```python
from build123d import *

# Parameters (mm, degrees)
F0_W          = 324
F0_H          = 18
F1_DEPTH      = 115
F2_DEPTH      = 130
F2_DEPTH_BACK = 10
F3_SIZE       = 8
F0_H_2        = 692
F4_DEPTH      = 4


with BuildPart() as f1:
    # F0 (on Top) → F1 (new body)
    with BuildSketch(Plane.XY):
        Polygon((162, 710), (162, 18), (180, 18), (180, 728), (162, 728), align=None)
        with Locations((0, 719)):
            Rectangle(F0_W, F0_H)
        Polygon((-180, 728), (-180, 18), (-162, 18), (-162, 710), (-162, 728), align=None)
    extrude(amount=F1_DEPTH)

    # F0 (on Top) → F2 (join, two sides)
    with BuildSketch(Plane.XY) as f2_sk:
        Polygon((-162, 18), (-180, 18), (-200, 18), (-200, 0), (200, 0), (200, 18), (180, 18), (162, 18), align=None)
    extrude(amount=F2_DEPTH)
    extrude(f2_sk.sketch, amount=-F2_DEPTH_BACK)

    # F3
    f3_edges = [f1.edges().sort_by_distance(p)[0] for p in [
        (0, 18, 130),
    ]]
    chamfer(f3_edges, length=F3_SIZE)

    # F0 (on Top) → F4 (join)
    with BuildSketch(Plane.XY):
        with Locations((0, 364)):
            Rectangle(F0_W, F0_H_2)
    extrude(amount=F4_DEPTH)


solid = f1.part
```
Part model, mm, in its own coordinate system. A direction names the side the tool comes from. Round coordinates to 2 decimals unless told otherwise and drop trailing zeros. Loops run counter-clockwise (first coordinate to the right, second up) from the corner with the lowest first, then second, coordinate; pieces in that order, holes last. Notation, with made-up numbers: (51, 5.5) -> (70, 5.5) arc R19 cw to (70, 25.5) -> close; hole circle Ø9 at (23, 35.5). An arc over 180 degrees is marked (long way). Use a Markdown table: item, result.
1) Cut at A-A, the plane z = 26. List the corners of the cut face in (x, y), and give its area (3 significant figures).
The answers:
| item | result |
|---|---|
| outline | (-200, 0) -> (200, 0) -> (200, 18) -> (180, 18) -> (180, 728) -> (-180, 728) -> (-180, 18) -> (-200, 18) -> close; hole (-162, 18) -> (162, 18) -> (162, 710) -> (-162, 710) -> close |
| area | 38,600 mm2 |
2) Drop flat-ended pins along their axis: pin 1 Ø10 at (x, y) = (100, 189) entering from -Z; pin 2 Ø1.5 at (x, y) = (-96.5, 480.5) entering from +Z; pin 3 Ø5 at (y, z) = (271, 91.5) entering from -X. Give the stop position or say it passes through.
The answers:
| item | result |
|---|---|
| pin 1 | stops at z = 0 |
| pin 2 | stops at z = 4 |
| pin 3 | stops at x = -180 |
3) Pull direction Y, two halves, no side cores. Call faces 1 (the flat face through (-3, 0, 61)), 2 (the flat face through (3, 18, 57)), 3 (the flat face through (-3, 378, 0)): pulls with the +Y half, pulls with the -Y half, needs draft (parallel to the pull), parting line crosses it, or undercut.
The answers:
| item | result |
|---|---|
| face 1 | pulls with the -Y half |
| face 2 | undercut |
| face 3 | needs draft |
4) Cut at C-C, the plane y = 51. List the corners of the cut face in (x, z), and give its area (3 significant figures).
The answers:
| item | result |
|---|---|
| outline | (-180, 0) -> (180, 0) -> (180, 115) -> (162, 115) -> (162, 4) -> (-162, 4) -> (-162, 115) -> (-180, 115) -> close |
| area | 5,440 mm2 |
5) Cut at B-B, the plane x = 7. List the corners of the cut face in (y, z), and give its area (3 significant figures).
The answers:
| item | result |
|---|---|
| outline | (0, -10) -> (18, -10) -> (18, 0) -> (728, 0) -> (728, 115) -> (710, 115) -> (710, 4) -> (18, 4) -> (18, 122) -> (10, 130) -> (0, 130) -> close |
| area | 7,330 mm2 |
6) Tool access for faces 4 (the flat face through (-174, 480, 115)), 5 (the flat face through (-180, 378, 57)), 6 (the flat face through (200, 9, 61)), 7 (the flat face through (180, 368, 57)), 8 (the flat face through (162, 369, 59)): list every direction of +Z, -Z, +X, -X, +Y, -Y with a clear straight run to the whole face (end or side of a thin tool).
The answers:
| item | result |
|---|---|
| face 4 | +Z, +X, -X, +Y |
| face 5 | +Z, -Z, -X, +Y |
| face 6 | +Z, -Z, +X, +Y, -Y |
| face 7 | +Z, -Z, +X, +Y |
| face 8 | +Z |
7) Probe line 1 (X direction, y = 531.5, z = 55); line 2 (Y direction, x = 118.5, z = 60); line 3 (Z direction, x = -177, y = 341.5). List the from-to ranges inside material, lowest first. Write a range as [from, to].
The answers:
| item | result |
|---|---|
| line 1 | x = [-180, -162], [162, 180] |
| line 2 | y = [0, 18], [710, 728] |
| line 3 | z = [0, 115] |
